Build history of the part. All positions in model axes, mm. A direction names the side the tool comes from. Coordinates: 2 decimals unless noted, no trailing zeros. Loops run counter-clockwise (first coordinate to the right, second up) from the corner with the lowest first, then second, coordinate; pieces in that order, holes last.
(1) Slice it at D-D (z = 8.75). Give the cut face in (x, y).
(2) Slice it at A-A (z = 7.5). Give the cut face in (x, y), and give its area (3 significant figures).
(3) Two-plate mould, pull along Z, no slides. Class faces 1 (the face through (19.94, 8.06, 8.04)), 2 (the face through (6, 8, 10)), 3 (the face through (7, 17.1, 7)): pulls with the +Z half, pulls with the -Z half, needs draft (parallel to the pull), parting line crosses it, or undercut.
(4) Tool access for faces 4 (the face through (9.15, 15, 7)), 5 (the face through (4.556, 9.365, 7.465)), 6 (the face through (6, 8, 5)), 7 (the face through (17.1, 5.1, 4.8)): list every direction of +Z, -Z, +X, -X, +Y, -Y with a clear straight run to the whole face (end or side of a thin tool).
(5) Flat gauge pins, fed straight in: P1, Ø5.5, axis at x = 3, y = 8.5, coming from the +Z side; P2, Ø3.5, axis at y = 14.5, z = 7, coming from the +X side; P3, Ø3, axis at y = 5, z = 5.5, coming from the +X side; P4, Ø2.5, axis at x = 3.75, y = 8.1, coming from the -Z side (1 decimal). Where does each tip first touch, or does it go through?
(6) Slice it at C-C (x = 4.25). Give the cut face in (y, z), and give its area (3 significant figures).
(7) Wall check: L1, parallel to X at y = 6.9, z = 7.5; L2, parallel to X at y = 8.1, z = 6.6; L3, parallel to Z at x = 4.75, y = 0.5. Give the ranges that are in metal, low to high.
(8) Slice it at B-B (y = 8.1). Give the cut face in (x, z), and give its area (3 significant figures).
from build123d import *
from build123d.topology import SkipClean

# Parameters (mm, degrees)
CROQUIS1_R              = 1.5
SALIENTE_EXTRUIR1_DEPTH = 15
CROQUIS2_R              = 2.5
CORTAR_EXTRUIR1_DEPTH   = 20
CORTAR_EXTRUIR2_START   = -22
CORTAR_EXTRUIR2_DEPTH   = 22
CROQUIS4_W              = 2.1
CROQUIS4_H              = 6
CORTAR_EXTRUIR4_DEPTH   = 10
REDONDEO1_R             = 1.5


with BuildPart() as part:
    # Croquis1 → Saliente-Extruir1 (new body)
    with BuildSketch(Plane.XY):
        with BuildLine():
            Line((11.25, 17.1), (11.25, 11.1))
            Line((11.25, 11.1), (23.75, 11.1))
            Line((23.75, 11.1), (23.75, 5.1))
            Line((23.75, 5.1), (11.25, 5.1))
            Line((11.25, 5.1), (11.25, -0.9))
            Line((11.25, -0.9), (5.75, -0.9))
            ThreePointArc((5.75, -0.9), (0.800252532, 1.150252532), (-1.25, 6.1))
            Line((-1.25, 6.1), (-1.25, 10.1))
            ThreePointArc((-1.25, 10.1), (0.800252532, 15.049747468), (5.75, 17.1))
            Line((5.75, 17.1), (11.25, 17.1))
        make_face()
        with Locations((3.75, 8.1)):
            Circle(CROQUIS1_R, mode=Mode.SUBTRACT)
    extrude(amount=SALIENTE_EXTRUIR1_DEPTH)

    # Croquis2 → Cortar-Extruir1 (cut)
    with BuildSketch(Plane(origin=(0, 0, 0), x_dir=(1, 0, 0), z_dir=(0, 1, 0))):
        with Locations(Location((17.5, -7.5, 0), (0, 0, 90))):
            Circle(CROQUIS2_R)
        with BuildLine():
            Line((17.5, -1.25), (11.25, 0))
            Line((11.25, 0), (11.126279301, 1.868603497))
            Line((11.126279301, 1.868603497), (29.663453957, 1.868603497))
            Line((29.663453957, 1.868603497), (29.663453957, -17.961269996))
            Line((29.663453957, -17.961269996), (11.25, -17.961269996))
            Line((11.25, -17.961269996), (11.25, -15))
            Line((11.25, -15), (17.5, -13.75))
            ThreePointArc((17.5, -13.75), (23.75, -7.5), (17.5, -1.25))
        make_face()
    extrude(amount=CORTAR_EXTRUIR1_DEPTH, mode=Mode.SUBTRACT)

    # Croquis3 → Cortar-Extruir2 (cut)
    with SkipClean():  # the faces are left unmerged after this step: merging them gives an invalid solid
        with BuildSketch(Plane(origin=(0, 17.1, 0), x_dir=(1, 0, 0), z_dir=(0, 1, 0)).offset(CORTAR_EXTRUIR2_START)):
            with BuildLine():
                Line((-4.130088798, -10), (9.25, -10))
                Line((9.25, -10), (14.284401529, -12.859330786))
                ThreePointArc((14.284401529, -12.859330786), (15.831665113, -13.523218301), (17.5, -13.75))
                Line((17.5, -13.75), (17.5, -15.581395259))
                Line((17.5, -15.581395259), (-4.130088798, -15.581395259))
                Line((-4.130088798, -15.581395259), (-4.130088798, -10))
            make_face()
            with BuildLine():
                Line((-3.464792336, -5), (9.25, -5))
                Line((9.25, -5), (14.284401529, -2.140669214))
                ThreePointArc((14.284401529, -2.140669214), (15.831665113, -1.476781699), (17.5, -1.25))
                Line((17.5, -1.25), (17.5, 1.677177667))
                Line((17.5, 1.677177667), (-3.464792336, 1.677177667))
                Line((-3.464792336, 1.677177667), (-3.464792336, -5))
            make_face()
        extrude(amount=CORTAR_EXTRUIR2_DEPTH, mode=Mode.SUBTRACT)

    # Croquis4 → Cortar-Extruir4 (cut, symmetric)
    with SkipClean():  # the faces are left unmerged after this step: merging them gives an invalid solid
        with BuildSketch(Plane.XY.offset(10)):
            with Locations((10.2, 14.1)):
                Rectangle(CROQUIS4_W, CROQUIS4_H)
            with Locations((10.2, 2.1)):
                Rectangle(CROQUIS4_W, CROQUIS4_H)
        extrude(amount=CORTAR_EXTRUIR4_DEPTH, both=True, mode=Mode.SUBTRACT)

    # Redondeo1
    # the kernel refuses this fillet: 1.5 mm, written as the material it adds along each edge
    with BuildSketch(Plane(origin=(9.15, 5.1, 1.25), x_dir=(0, -1, 0), z_dir=(0, 0, 1))) as redondeo1_piece_1_section:
        with BuildLine():
            CenterArc((REDONDEO1_R, REDONDEO1_R), REDONDEO1_R, 180, 90)
            Line((0, REDONDEO1_R), (0, 0))
            Line((0, 0), (REDONDEO1_R, 0))
        make_face()
    redondeo1_piece_1 = extrude(amount=8.75, mode=Mode.PRIVATE)
    redondeo1_piece_1 = split(redondeo1_piece_1, bisect_by=Plane(origin=(9.866987005, 4.973706672, 5), z_dir=(0, 0, -1)), keep=Keep.TOP, mode=Mode.PRIVATE)
    redondeo1_piece_1 = split(redondeo1_piece_1, bisect_by=Plane(origin=(9.791745369, 4.973706672, 4.692311151), z_dir=(0.49386255985599625, 0, 0.8695399772135164)), keep=Keep.TOP, mode=Mode.PRIVATE)
    add(redondeo1_piece_1)
    with BuildSketch(Plane(origin=(9.15, 5.1, 5), x_dir=(0, -1, 0), z_dir=(0, 0, 1))) as redondeo1_piece_2_section:
        with BuildLine():
            CenterArc((REDONDEO1_R, REDONDEO1_R), REDONDEO1_R, 180, 90)
            Line((0, REDONDEO1_R), (0, 0))
            Line((0, 0), (REDONDEO1_R, 0))
        make_face()
    redondeo1_piece_2 = extrude(amount=5, mode=Mode.PRIVATE)
    redondeo1_piece_2 = split(redondeo1_piece_2, bisect_by=Plane(origin=(9.170637547, 4.440228568, 5.045074574), z_dir=(-0.49386255985599625, 0, -0.8695399772135164)), keep=Keep.TOP, mode=Mode.PRIVATE)
    add(redondeo1_piece_2)
    with BuildSketch(Plane(origin=(9.15, 5.1, 5), x_dir=(0, -1, 0), z_dir=(0, 0, 1))) as redondeo1_piece_3_section:
        with BuildLine():
            CenterArc((REDONDEO1_R, REDONDEO1_R), REDONDEO1_R, 180, 90)
            Line((0, REDONDEO1_R), (0, 0))
            Line((0, 0), (REDONDEO1_R, 0))
        make_face()
    redondeo1_piece_3 = extrude(amount=5, mode=Mode.PRIVATE)
    redondeo1_piece_3 = split(redondeo1_piece_3, bisect_by=Plane(origin=(8.358711998, 4.761869179, 9.493785466), z_dir=(0.49386255985599636, 0, -0.8695399772135163)), keep=Keep.TOP, mode=Mode.PRIVATE)
    redondeo1_piece_3 = split(redondeo1_piece_3, bisect_by=Plane(origin=(8.358711998, 4.761869179, 5.506214534), z_dir=(0.49386255985599625, 0, 0.8695399772135164)), keep=Keep.TOP, mode=Mode.PRIVATE)
    add(redondeo1_piece_3)
    with BuildSketch(Plane(origin=(9.15, 5.1, 5), x_dir=(0, -1, 0), z_dir=(0, 0, 1))) as redondeo1_piece_4_section:
        with BuildLine():
            CenterArc((REDONDEO1_R, REDONDEO1_R), REDONDEO1_R, 180, 90)
            Line((0, REDONDEO1_R), (0, 0))
            Line((0, 0), (REDONDEO1_R, 0))
        make_face()
    redondeo1_piece_4 = extrude(amount=8.75, mode=Mode.PRIVATE)
    redondeo1_piece_4 = split(redondeo1_piece_4, bisect_by=Plane(origin=(9.866987005, 4.973706672, 10), z_dir=(0, 0, 1)), keep=Keep.TOP, mode=Mode.PRIVATE)
    redondeo1_piece_4 = split(redondeo1_piece_4, bisect_by=Plane(origin=(9.791745369, 4.973706672, 10.307688849), z_dir=(0.49386255985599636, 0, -0.8695399772135163)), keep=Keep.TOP, mode=Mode.PRIVATE)
    add(redondeo1_piece_4)
    with BuildSketch(Plane(origin=(9.15, 5.1, 5), x_dir=(0, -1, 0), z_dir=(0, 0, 1))) as redondeo1_piece_5_section:
        with BuildLine():
            CenterArc((REDONDEO1_R, REDONDEO1_R), REDONDEO1_R, 180, 90)
            Line((0, REDONDEO1_R), (0, 0))
            Line((0, 0), (REDONDEO1_R, 0))
        make_face()
    redondeo1_piece_5 = extrude(amount=5, mode=Mode.PRIVATE)
    redondeo1_piece_5 = split(redondeo1_piece_5, bisect_by=Plane(origin=(9.170637547, 4.440228568, 9.954925426), z_dir=(-0.49386255985599636, 0, 0.8695399772135163)), keep=Keep.TOP, mode=Mode.PRIVATE)
    add(redondeo1_piece_5)
    with BuildSketch(Plane(origin=(9.15, 11.1, 5), x_dir=(1, 0, 0), z_dir=(0, 0, 1))) as redondeo1_piece_6_section:
        with BuildLine():
            CenterArc((REDONDEO1_R, REDONDEO1_R), REDONDEO1_R, 180, 90)
            Line((0, REDONDEO1_R), (0, 0))
            Line((0, 0), (REDONDEO1_R, 0))
        make_face()
    redondeo1_piece_6 = extrude(amount=5, mode=Mode.PRIVATE)
    redondeo1_piece_6 = split(redondeo1_piece_6, bisect_by=Plane(origin=(9.17063755, 11.759771469, 5.045074573), z_dir=(-0.49386255985599625, 0, -0.8695399772135164)), keep=Keep.TOP, mode=Mode.PRIVATE)
    add(redondeo1_piece_6)
    with BuildSketch(Plane(origin=(9.15, 11.1, 1.25), x_dir=(1, 0, 0), z_dir=(0, 0, 1))) as redondeo1_piece_7_section:
        with BuildLine():
            CenterArc((REDONDEO1_R, REDONDEO1_R), REDONDEO1_R, 180, 90)
            Line((0, REDONDEO1_R), (0, 0))
            Line((0, 0), (REDONDEO1_R, 0))
        make_face()
    redondeo1_piece_7 = extrude(amount=8.75, mode=Mode.PRIVATE)
    redondeo1_piece_7 = split(redondeo1_piece_7, bisect_by=Plane(origin=(9.866987013, 11.226293308, 5), z_dir=(0, 0, -1)), keep=Keep.TOP, mode=Mode.PRIVATE)
    redondeo1_piece_7 = split(redondeo1_piece_7, bisect_by=Plane(origin=(9.791745378, 11.226293308, 4.692311146), z_dir=(0.49386255985599625, 0, 0.8695399772135164)), keep=Keep.TOP, mode=Mode.PRIVATE)
    add(redondeo1_piece_7)
    with BuildSketch(Plane(origin=(9.15, 11.1, 5), x_dir=(1, 0, 0), z_dir=(0, 0, 1))) as redondeo1_piece_8_section:
        with BuildLine():
            CenterArc((REDONDEO1_R, REDONDEO1_R), REDONDEO1_R, 180, 90)
            Line((0, REDONDEO1_R), (0, 0))
            Line((0, 0), (REDONDEO1_R, 0))
        make_face()
    redondeo1_piece_8 = extrude(amount=5, mode=Mode.PRIVATE)
    redondeo1_piece_8 = split(redondeo1_piece_8, bisect_by=Plane(origin=(8.358711999, 11.438130822, 5.506214534), z_dir=(0.49386255985599625, 0, 0.8695399772135164)), keep=Keep.TOP, mode=Mode.PRIVATE)
    redondeo1_piece_8 = split(redondeo1_piece_8, bisect_by=Plane(origin=(8.358711999, 11.438130822, 9.493785466), z_dir=(0.49386255985599636, 0, -0.8695399772135163)), keep=Keep.TOP, mode=Mode.PRIVATE)
    add(redondeo1_piece_8)
    with BuildSketch(Plane(origin=(9.15, 11.1, 5), x_dir=(1, 0, 0), z_dir=(0, 0, 1))) as redondeo1_piece_9_section:
        with BuildLine():
            CenterArc((REDONDEO1_R, REDONDEO1_R), REDONDEO1_R, 180, 90)
            Line((0, REDONDEO1_R), (0, 0))
            Line((0, 0), (REDONDEO1_R, 0))
        make_face()
    redondeo1_piece_9 = extrude(amount=5, mode=Mode.PRIVATE)
    redondeo1_piece_9 = split(redondeo1_piece_9, bisect_by=Plane(origin=(9.17063755, 11.759771469, 9.954925427), z_dir=(-0.49386255985599636, 0, 0.8695399772135163)), keep=Keep.TOP, mode=Mode.PRIVATE)
    add(redondeo1_piece_9)
    with BuildSketch(Plane(origin=(9.15, 11.1, 5), x_dir=(1, 0, 0), z_dir=(0, 0, 1))) as redondeo1_piece_10_section:
        with BuildLine():
            CenterArc((REDONDEO1_R, REDONDEO1_R), REDONDEO1_R, 180, 90)
            Line((0, REDONDEO1_R), (0, 0))
            Line((0, 0), (REDONDEO1_R, 0))
        make_face()
    redondeo1_piece_10 = extrude(amount=8.75, mode=Mode.PRIVATE)
    redondeo1_piece_10 = split(redondeo1_piece_10, bisect_by=Plane(origin=(9.866987013, 11.226293308, 10), z_dir=(0, 0, 1)), keep=Keep.TOP, mode=Mode.PRIVATE)
    redondeo1_piece_10 = split(redondeo1_piece_10, bisect_by=Plane(origin=(9.791745378, 11.226293308, 10.307688854), z_dir=(0.49386255985599636, 0, -0.8695399772135163)), keep=Keep.TOP, mode=Mode.PRIVATE)
    add(redondeo1_piece_10)


solid = part.part
Response values:
1. outline: (-1.25, 6.1) arc R7 ccw to (5.75, -0.9) - (9.15, -0.9) - (9.15, 3.6) arc R1.5 cw to (10.65, 5.1) - (15.33, 5.1) - (15.33, 11.1) - (10.65, 11.1) arc R1.5 cw to (9.15, 12.6) - (9.15, 17.1) - (5.75, 17.1) arc R7 ccw to (-1.25, 10.1) - close; (19.67, 5.1) - (23.62, 5.1) - (23.62, 11.1) - (19.67, 11.1) - close; hole circle Ø3 at (3.75, 8.1)
2. outline: (-1.25, 6.1) arc R7 ccw to (5.75, -0.9) - (9.15, -0.9) - (9.15, 3.6) arc R1.5 cw to (10.65, 5.1) - (15, 5.1) - (15, 11.1) - (10.65, 11.1) arc R1.5 cw to (9.15, 12.6) - (9.15, 17.1) - (5.75, 17.1) arc R7 ccw to (-1.25, 10.1) - close; (20, 5.1) - (23.75, 5.1) - (23.75, 11.1) - (20, 11.1) - close; hole circle Ø3 at (3.75, 8.1)
2. area: 218 mm2
3. face 1: undercut
3. face 2: pulls with the +Z half
3. face 3: needs draft
4. face 4: +Z, -Z, +X, +Y
4. face 5: +Z, -Z
4. face 6: -Z, -X, +Y, -Y
4. face 7: +Z, -Z, +X, -Y
5. P1: stops at z = 10
5. P2: stops at x = 9.15
5. P3: stops at x = 23.73
5. P4: passes through
6. outline: (-0.74, 5) - (6.69, 5) - (6.69, 10) - (-0.74, 10) - close; (9.51, 5) - (16.94, 5) - (16.94, 10) - (9.51, 10) - close
6. area: 74.2 mm2
7. L1: x = -1.25 to 2.85, 4.65 to 15, 20 to 23.75
7. L2: x = -1.25 to 2.25, 5.25 to 15.17, 19.83 to 23.68
7. L3: z = 5 to 10
8. outline: (-1.25, 5) - (2.25, 5) - (2.25, 10) - (-1.25, 10) - close; (5.25, 5) - (9.25, 5) - (14.28, 2.14) arc R6.25 ccw (long way) to (14.28, 12.86) - (9.25, 10) - (5.25, 10) - close; hole circle Ø5 at (17.5, 7.5)
8. area: 157 mm2
